from build123d import *

# Parameters (mm, degrees)
BOSS_EXTRUDE2_DEPTH = 5
SKETCH2_W           = 24
SKETCH2_H           = 12.4
CUT_EXTRUDE1_DEPTH  = 5
SKETCH3_R           = 1.2
CUT_EXTRUDE2_DEPTH  = 5
SKETCH5_R           = 0.975
CUT_EXTRUDE3_DEPTH  = 10
SKETCH6_R           = 17.5
CUT_EXTRUDE4_DEPTH  = 10
SKETCH8_R           = 1.6
CUT_EXTRUDE5_DEPTH  = 10
BOSS_EXTRUDE3_DEPTH = 17.7
SKETCH12_R          = 1.2
CUT_EXTRUDE6_DEPTH  = 5


with BuildPart() as part:
    # Sketch1 → Boss-Extrude2 (new body)
    with BuildSketch(Plane.XY):
        with BuildLine():
            Line((-90, -50), (90, -50))
            ThreePointArc((90, -50), (100.606601718, -45.606601718), (105, -35))
            Line((105, -35), (105, 35))
            ThreePointArc((105, 35), (100.606601718, 45.606601718), (90, 50))
            Line((90, 50), (-90, 50))
            ThreePointArc((-90, 50), (-100.606601718, 45.606601718), (-105, 35))
            Line((-105, 35), (-105, -35))
            ThreePointArc((-105, -35), (-100.606601718, -45.606601718), (-90, -50))
        make_face()
    extrude(amount=BOSS_EXTRUDE2_DEPTH)

    # Sketch2 → Cut-Extrude1 (cut)
    with BuildSketch(Plane.XY.offset(5)):
        with Locations((63, -43.8)):
            Rectangle(SKETCH2_W, SKETCH2_H)
        with Locations((-63, 43.8)):
            Rectangle(SKETCH2_W, SKETCH2_H)
        with Locations((0, 43.8)):
            Rectangle(SKETCH2_W, SKETCH2_H)
        with Locations((63, 43.8)):
            Rectangle(SKETCH2_W, SKETCH2_H)
        with Locations((0, -43.8)):
            Rectangle(SKETCH2_W, SKETCH2_H)
        with Locations((-63, -43.8)):
            Rectangle(SKETCH2_W, SKETCH2_H)
    extrude(amount=-CUT_EXTRUDE1_DEPTH, mode=Mode.SUBTRACT)

    # Sketch3 → Cut-Extrude2 (cut)
    with BuildSketch(Plane.XY.offset(5)):
        with Locations((-76.8, 43.8)):
            Circle(SKETCH3_R)
        with Locations((-49.2, 43.8)):
            Circle(SKETCH3_R)
        with Locations((-13.8, 43.8)):
            Circle(SKETCH3_R)
        with Locations((13.8, 43.8)):
            Circle(SKETCH3_R)
        with Locations((49.2, 43.8)):
            Circle(SKETCH3_R)
        with Locations((76.8, 43.8)):
            Circle(SKETCH3_R)
        with Locations((-76.8, -43.8)):
            Circle(SKETCH3_R)
        with Locations((-49.2, -43.8)):
            Circle(SKETCH3_R)
        with Locations((-13.8, -43.8)):
            Circle(SKETCH3_R)
        with Locations((13.8, -43.8)):
            Circle(SKETCH3_R)
        with Locations((49.2, -43.8)):
            Circle(SKETCH3_R)
        with Locations((76.8, -43.8)):
            Circle(SKETCH3_R)
    extrude(amount=-CUT_EXTRUDE2_DEPTH, mode=Mode.SUBTRACT)

    # Sketch5 → Cut-Extrude3 (cut)
    with BuildSketch(Plane.XY.offset(5)):
        with Locations((-36.75, 43.360200931)):
            Circle(SKETCH5_R)
        with Locations((26.25, 43.360200931)):
            Circle(SKETCH5_R)
        with Locations((26.25, -43.360200931)):
            Circle(SKETCH5_R)
        with Locations((-36.75, -43.360200931)):
            Circle(SKETCH5_R)
        with Locations((-99.75, 43.360200931)):
            Circle(SKETCH5_R)
        with Locations((-99.75, -43.360200931)):
            Circle(SKETCH5_R)
    extrude(amount=-CUT_EXTRUDE3_DEPTH, mode=Mode.SUBTRACT)

    # Sketch6 → Cut-Extrude4 (cut)
    with BuildSketch(Plane.XY.offset(5)):
        with Locations((-105, 0)):
            Circle(SKETCH6_R)
    extrude(amount=-CUT_EXTRUDE4_DEPTH, mode=Mode.SUBTRACT)

    # Sketch8 → Cut-Extrude5 (cut)
    with BuildSketch(Plane(origin=(0, 0, 0), x_dir=(-1, 0, 0), z_dir=(0, 0, -1))):
        with Locations((31.97, 24.11)):
            Circle(SKETCH8_R)
        with Locations((38.33, -24.11)):
            Circle(SKETCH8_R)
        with Locations((7.88, 8.88)):
            Circle(SKETCH8_R)
        with Locations((7.88, -19.03)):
            Circle(SKETCH8_R)
        with Locations((-42.91, 24.11)):
            Circle(SKETCH8_R)
        with Locations((-44.24, -24.11)):
            Circle(SKETCH8_R)
        with Locations((-73.65, 18)):
            Circle(SKETCH8_R)
        with Locations((48.35, 15)):
            Circle(SKETCH8_R)
        with Locations((-73.65, -18)):
            Circle(SKETCH8_R)
        with Locations((48.35, -15)):
            Circle(SKETCH8_R)
        with Locations((-33.65, 32)):
            Circle(SKETCH8_R)
        with Locations((16.35, 32)):
            Circle(SKETCH8_R)
        with Locations((-33.65, -32)):
            Circle(SKETCH8_R)
        with Locations((16.35, -32)):
            Circle(SKETCH8_R)
    extrude(amount=-CUT_EXTRUDE5_DEPTH, mode=Mode.SUBTRACT)

    # Sketch10 → Boss-Extrude3 (add)
    with BuildSketch(Plane(origin=(0, 0, 0), x_dir=(-1, 0, 0), z_dir=(0, 0, -1))):
        Polygon((71.290147782, 0), (71.290147782, -11.5), (58.890147782, -11.5), (58.890147782, 11.5), (71.290147782, 11.5), (71.290147782, 16.5), (53.890147782, 16.5), (53.890147782, -16.5), (76.290147782, -16.5), (76.290147782, 0), align=None)
    extrude(amount=BOSS_EXTRUDE3_DEPTH)

    # Sketch12 → Cut-Extrude6 (cut)
    with BuildSketch(Plane(origin=(0, 0, -17.7), x_dir=(-1, 0, 0), z_dir=(0, 0, -1))):
        with Locations((65.090147782, -13.8)):
            Circle(SKETCH12_R)
        with Locations((65.090147782, 13.8)):
            Circle(SKETCH12_R)
    extrude(amount=-CUT_EXTRUDE6_DEPTH, mode=Mode.SUBTRACT)


solid = part.part
For this review, take the finished solid that the model builds, in its own axes (mm). A direction names the side the tool comes from. Round coordinates to 2 decimals unless told otherwise and drop trailing zeros. Write each loop counter-clockwise with the first axis right and the second up, starting at its lowest first coordinate (ties: lowest second). Pieces come first, ordered by that corner, then holes. Notation, with made-up numbers: M 24,42.5 L 41,42.5 A31 cw 41,67.5 Z; hole C 8.5,55.25 d8. An arc over 180 degrees is marked long. Write item = value, one per line. Start each with the question number.
(1) We need section C-C (x = 56). Give the boundary of the cut face in (y, z).
(2) The part is to be moulded in two halves that separate along X. For faces 1 (the face through (100.49, -45.72, 2.46)), 2 (the face through (-87.504, -0.385, 2.535)), 3 (the face through (-51, -44, 3)), 4 (the face through (-65, -16.5, -9)), say which applies: +X half, -X half, draft (parallel to the pull), parting line (faces both ways), or undercut.
(3) For line 1 along Y through (x, z) = (33.65, 3.05); line 2 along Y through (x, z) = (73.65, 3.8); line 3 along Y through (x, z) = (-38.33, 2), list the stretches that pass through material, from the lowest coordinate up.
(4) For faces 5 (the face through (-53.89, 0, -9)), 6 (the face through (-76.29, -8, -9)), 7 (the face through (0, 37.6, 3)), list the 3-axis set-ups (+Z, -Z, +X, -X, +Y, -Y) from which the entire face can be reached by the end or side of a thin tool; tool diameter is ignored.
(5) We need section B-B (y = -40). Give the boundary of the cut face in (x, z).
(6) We need section A-A (z = -14.75). Give the boundary of the cut face in (x, y), then the cut area to 3 significant figures.
(7) Clearance check with flat-ended pins moving along their axes: pin 1 Ø5 at (x, z) = (-58.5, -7.5) entering from +Y; pin 2 Ø10 at (x, z) = (-62.5, -5.5) entering from -Y; pin 3 Ø5 at (x, z) = (70, 2.5) entering from +Y. State where each tip first meets the part, or that it passes through.
Results found:
q1.outline = M -37.6,0 L 37.6,0 L 37.6,5 L -37.6,5 Z
q2.face_1 = +X half
q2.face_2 = -X half
q2.face_3 = undercut
q2.face_4 = draft
q3.line_1 = -50 to -33.6, -30.4 to 30.4, 33.6 to 50
q3.line_2 = -37.6 to -19.6, -16.4 to 16.4, 19.6 to 37.6
q3.line_3 = -50 to -25.71, -22.51 to 50
q4.face_5 = -Z, +X, +Y, -Y
q4.face_6 = -Z, -X, +Y, -Y
q4.face_7 = +Z, -Z, +Y
q5.outline = M -104.14,0 L -75,0 L -75,5 L -104.14,5 Z; M -51,0 L -12,0 L -12,5 L -51,5 Z; M 12,0 L 51,0 L 51,5 L 12,5 Z; M 75,0 L 104.14,0 L 104.14,5 L 75,5 Z
q6.outline = M -76.29,-16.5 L -53.89,-16.5 L -53.89,16.5 L -71.29,16.5 L -71.29,11.5 L -58.89,11.5 L -58.89,-11.5 L -71.29,-11.5 L -71.29,0 L -76.29,0 Z; hole C -65.09,-13.8 d2.4; hole C -65.09,13.8 d2.4
q6.area = 362 mm²
q7.pin_1 = 16.5
q7.pin_2 = -16.5
q7.pin_3 = 37.6
